Design review of the part built by this model. Coordinates are the model's own, in mm. Face numbers are marked on the shaded views. A direction names the side the tool comes from. Give positions to 0.01 mm unless a question says otherwise; leave off trailing zeros. Write each loop counter-clockwise with the first axis right and the second up, starting at its lowest first coordinate (ties: lowest second). Pieces come first, ordered by that corner, then holes. Notation, with made-up numbers: M 50,80 L 94,80 A18 ccw 94,115 Z; hole C 89,40 d2. An arc over 180 degrees is marked long. One line per item, written item: value. Start each with the question number.
```python
from build123d import *

# Parameters (mm, degrees)
SKETCH027_R     = 1.7
PAD016_DEPTH    = 3
PAD017_DEPTH    = 3
SKETCH029_R     = 1.7
POCKET007_DEPTH = 26.619333
PAD018_DEPTH    = 5
PAD019_DEPTH    = 4
POCKET011_DEPTH = 31.8
POCKET012_DEPTH = 80.219333


with BuildPart() as part:
    # Sketch027 (on Face4 of Binder003) → Pad016 (new body)
    with BuildSketch(Plane(origin=(0, 0, -8.7), x_dir=(1, 0, 0), z_dir=(0, 0, -1))):
        Polygon((63, -0.2), (63, -10.2), (14.581667, -73.3), (126.418333, -73.3), (102.8, -42.519989), (102.8, -0.2), align=None)
        with Locations((70.5, -13.2)):
            Circle(SKETCH027_R, mode=Mode.SUBTRACT)
        with Locations((107.8, -60.3)):
            Circle(SKETCH027_R, mode=Mode.SUBTRACT)
        with Locations((33.2, -60.3)):
            Circle(SKETCH027_R, mode=Mode.SUBTRACT)
    extrude(amount=PAD016_DEPTH)

    # Sketch028 (on Face6 of Pad016) → Pad017 (join)
    with BuildSketch(Plane.YZ.offset(102.8)):
        Polygon((0.2, -11.7), (48.475, -95.314753), (83.116016, -75.314753), (53.116016, -23.353229), (73.3, -11.7), align=None)
    extrude(amount=-PAD017_DEPTH)

    # Sketch029 (on Face14 of Pad017) → Pocket007 (cut, through all)
    with BuildSketch(Plane(origin=(99.8, 0, 0), x_dir=(0, -1, 0), z_dir=(-1, 0, 0))):
        with Locations((-51.846002, -81.821499)):
            Circle(SKETCH029_R)
        with Locations((-41.846002, -64.500991)):
            Circle(SKETCH029_R)
        with Locations((-64.16651, -63.161245)):
            Circle(SKETCH029_R)
    extrude(amount=-POCKET007_DEPTH, mode=Mode.SUBTRACT)

    # Sketch030 (on Face14 of Pocket007) → Pad018 (join)
    with BuildSketch(Plane(origin=(99.8, 0, 0), x_dir=(0, -1, 0), z_dir=(-1, 0, 0))):
        Polygon((-0.2, -11.7), (-48.475, -95.314753), (-51.073076, -93.814753), (-3.664102, -11.7), align=None)
        Polygon((-42.92392, -11.7), (-80.51794, -76.814753), (-83.116016, -75.314753), (-53.116016, -23.353229), (-73.3, -11.7), align=None)
        Polygon((-21.56196, -11.7), (-64.49647, -86.064753), (-67.094546, -84.564753), (-25.026062, -11.7), align=None)
    extrude(amount=PAD018_DEPTH)

    # Sketch031 (on Face5 of Pad018) → Pad019 (join)
    with BuildSketch(Plane(origin=(0, 0, -11.7), x_dir=(1, 0, 0), z_dir=(0, 0, -1))):
        Polygon((94.8, -3.664102), (66, -3.664102), (66, -11.218363), (20.665065, -70.3), (57.401987, -70.3), (94.8, -21.56196), (94.8, -25.026062), (60.060085, -70.3), (94.8, -70.3), (94.8, -73.3), (14.581667, -73.3), (63, -10.2), (63, -0.2), (94.8, -0.2), align=None)
    extrude(amount=PAD019_DEPTH)

    # Sketch036 (on Face16 of Pad019) → Pocket011 (cut)
    with BuildSketch(Plane.YZ.offset(94.8)):
        Polygon((2.509401, -15.7), (0.2, -15.7), (0.2, -11.7), align=None)
        Polygon((23.871361, -15.7), (21.56196, -11.7), (21.56196, -15.7), align=None)
    extrude(amount=-POCKET011_DEPTH, mode=Mode.SUBTRACT)

    # Sketch037 (on Face30 of Pocket011) → Pocket012 (cut, through all)
    with BuildSketch(Plane.YZ.offset(94.8)):
        Polygon((73.3, -11.7), (73.3, -15.7), (66.371797, -15.7), align=None)
    extrude(amount=-POCKET012_DEPTH, mode=Mode.SUBTRACT)


solid = part.part
```
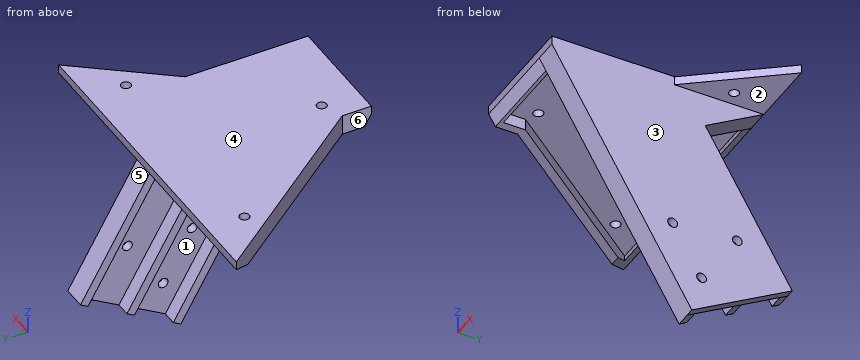
Q1. Take a section at A-A, the plane x = 33.2. Give the boundary of the cut face in (y, z).
Q2. Machinability: for the marked faces 4, 5 and 6, which of the approach directions +Z, -Z, +X, -X, +Y, -Y give a long, thin tool a straight path to every point of the face, cutting with its end or side? Answer none if there is none.
Q3. Take a section at C-C, the plane y = 60.3. State how many separate pieces and enclosed holes the cut face has, then the cut area to 3 significant figures.
Q4. For P1, Ø25, axis at y = 25.5, z = -62.5, coming from the +X side; P2, Ø2.5, axis at y = 41.85, z = -64.5, coming from the +X side; P3, Ø10, axis at y = 53.5, z = -25.5, coming from the -X side; P4, Ø2, axis at x = 75, z = -13.5, coming from the +Y side, all flat-tipped, find the tip position at first contact; note any pin that passes through.
Q5. Take a section at D-D, the plane x = 74. Give the boundary of the cut face in (y, z), then the cut area to 3 significant figures.
Q6. Wall thickness on line 1 (X direction, y = 60.3, z = -10.15); line 2 (Y direction, x = 78.5, z = -13); line 3 (Z direction, x = 24.5, y = 61): over which ranges is each line inside the solid? List them lowest first. Write a range as from..to.
Q7. The part is to be moulded in two halves that separate along Z. For the marked faces 1, 2 and 3, say which applies: pulls with the +Z half, pulls with the -Z half, needs draft (parallel to the pull), parting line crosses it, or undercut.
Q8. Take a section at B-B, the plane y = 13.2. Give the boundary of the cut face in (x, z).
Results list:
1. outline: M 49.04,-15.7 L 53.96,-15.7 L 53.96,-11.7 L 58.6,-11.7 L 58.6,-8.7 L 49.04,-8.7 Z; M 62,-11.7 L 70.3,-11.7 L 70.3,-13.43 L 73.3,-11.7 L 73.3,-8.7 L 62,-8.7 Z
2. face 4: +Z, +X, -X, +Y, -Y
2. face 5: +X, -X, +Y
2. face 6: +Z, -Z, -X, -Y
3. separate pieces: 4
3. enclosed holes: 0
3. area: 559 mm^2
4. P1: stops at x = 102.8
4. P2: passes through
4. P3: stops at x = 94.8
4. P4: stops at y = 71.91
5. outline: M 0.2,-11.7 L 2.51,-15.7 L 3.66,-15.7 L 3.66,-11.7 L 48.67,-11.7 L 48.67,-15.7 L 52.13,-15.7 L 52.13,-11.7 L 70.3,-11.7 L 70.3,-13.43 L 73.3,-11.7 L 73.3,-8.7 L 0.2,-8.7 Z
5. area: 245 mm^2
6. line 1: x = 24.56..31.5, 34.9..106.1, 109.5..116.44
6. line 2: y = 0.95..3.66, 42.8..46.27, 70.3..71.05
6. line 3: z = -15.7..-8.7
7. face 1: undercut
7. face 2: pulls with the -Z half
7. face 3: needs draft
8. outline: M 60.7,-15.7 L 64.48,-15.7 L 64.48,-11.7 L 68.8,-11.7 L 68.8,-8.7 L 60.7,-8.7 Z; M 72.2,-11.7 L 99.8,-11.7 L 99.8,-28.22 L 94.8,-28.22 L 94.8,-34.22 L 102.8,-34.22 L 102.8,-8.7 L 72.2,-8.7 Z
